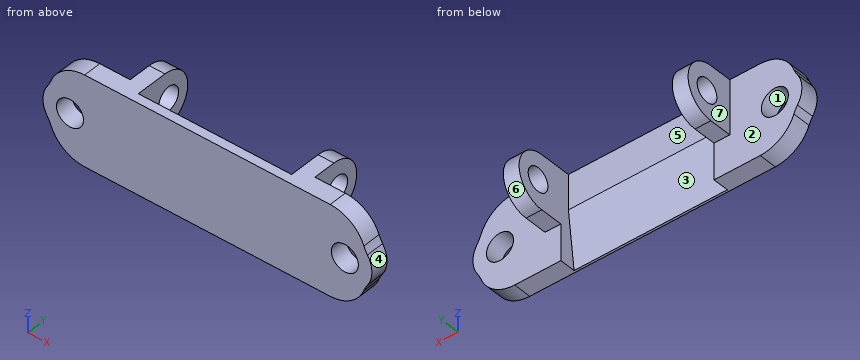
from build123d import *

# Parameters (mm, degrees)
BOSS_EXTRUDE1_DEPTH             = 4
CUT_EXTRUDE1_DEPTH              = 34
BOSS_EXTRUDE2_DEPTH             = 3.5
F_5_2_5_2_DIAMETER_HOLE1_REACH  = 64.241
F_5_2_5_2_DIAMETER_HOLE1_BORE_R = 2.6
F_6_0_6_DIAMETER_HOLE1_D        = 6
F_6_0_6_DIAMETER_HOLE1_DEPTH    = 15


with BuildPart() as part:
    # Sketch1 → Boss-Extrude1 (new body)
    with BuildSketch(Plane(origin=(0, 4, 0), x_dir=(1, 0, 0), z_dir=(0, 1, 0))):
        with BuildLine():
            Line((7.753999476, 0), (62.246000524, 0))
            ThreePointArc((62.246000524, 0), (66.787860981, 1.414295513), (69.723838222, 5.157124101))
            ThreePointArc((69.723838222, 5.157124101), (70.077199101, 5.953180748), (70.515003965, 6.706106372))
            ThreePointArc((70.515003965, 6.706106372), (71.5, 10), (70.515003965, 13.293893628))
            ThreePointArc((70.515003965, 13.293893628), (70.077199101, 14.046819252), (69.723838222, 14.842875899))
            ThreePointArc((69.723838222, 14.842875899), (66.787860981, 18.585704487), (62.246000524, 20))
            Line((62.246000524, 20), (52, 20))
            add(Edge.make_bspline(
                [(18, 20), (29.333333333, 20), (40.666666667, 20), (52, 20)],
                knots=[0, 0, 0, 0, 1, 1, 1, 1], degree=3))
            Line((18, 20), (7.753999476, 20))
            ThreePointArc((7.753999476, 20), (3.212139019, 18.585704487), (0.276161778, 14.842875899))
            ThreePointArc((0.276161778, 14.842875899), (-0.077199101, 14.046819252), (-0.515003965, 13.293893628))
            ThreePointArc((-0.515003965, 13.293893628), (-1.5, 10), (-0.515003965, 6.706106372))
            ThreePointArc((-0.515003965, 6.706106372), (-0.077199101, 5.953180748), (0.276161778, 5.157124101))
            ThreePointArc((0.276161778, 5.157124101), (3.212139019, 1.414295513), (7.753999476, 0))
        make_face()
    extrude(amount=-BOSS_EXTRUDE1_DEPTH)

    # Sketch2 → Cut-Extrude1 (cut)
    with BuildSketch(Plane(origin=(18, 0, 0), x_dir=(0, -1, 0), z_dir=(-1, 0, 0))):
        Polygon((-2, 0), (-4, 0), (-4, -20), (-0.499398694, -20), (-2, -7.707188193), align=None)
    extrude(amount=-CUT_EXTRUDE1_DEPTH, mode=Mode.SUBTRACT)

    # Sketch3 → Boss-Extrude2 (add)
    with BuildSketch(Plane(origin=(18, 0, 0), x_dir=(0, 0, -1), z_dir=(1, 0, 0))):
        with BuildLine():
            Line((0, 4), (12, 4))
            Line((12, 4), (12, 9))
            ThreePointArc((12, 9), (6, 15), (0, 9))
            Line((0, 9), (0, 4))
        make_face()
    boss_extrude2 = extrude(amount=-BOSS_EXTRUDE2_DEPTH)

    # Mirror1: Boss-Extrude2 across plane
    add(boss_extrude2.mirror(Plane.ZY.offset(-35)))

    # Ø5.2 (5.2) Diameter Hole1 bore → Ø5.2 (5.2) Diameter Hole1 (cut, up to next)
    with BuildSketch(Plane.ZY.offset(-14.5), mode=Mode.PRIVATE) as f_5_2_5_2_diameter_hole1_sk1:
        with Locations((-6, 10)):
            Circle(F_5_2_5_2_DIAMETER_HOLE1_BORE_R)
    f_5_2_5_2_diameter_hole1_tool1 = extrude(f_5_2_5_2_diameter_hole1_sk1.sketch, amount=-F_5_2_5_2_DIAMETER_HOLE1_REACH, mode=Mode.PRIVATE) & part.part
    f_5_2_5_2_diameter_hole1 = f_5_2_5_2_diameter_hole1_tool1.solids().sort_by_distance((14.5, 10, -6))[0]
    add(f_5_2_5_2_diameter_hole1, mode=Mode.SUBTRACT)

    # Ø6.0 (6) Diameter Hole1
    with Locations(Plane(origin=(0, 0, 0), x_dir=(-1, 0, 0), z_dir=(0, -1, 0))):
        with Locations((-4.5, 10)):
            f_6_0_6_diameter_hole1 = Hole(F_6_0_6_DIAMETER_HOLE1_D / 2, depth=F_6_0_6_DIAMETER_HOLE1_DEPTH)

    # Mirror2: Ø5.2 (5.2) Diameter Hole1, Ø6.0 (6) Diameter Hole1 across plane
    add(f_5_2_5_2_diameter_hole1.mirror(Plane.ZY.offset(-35)), mode=Mode.SUBTRACT)
    add(f_6_0_6_diameter_hole1.mirror(Plane.ZY.offset(-35)), mode=Mode.SUBTRACT)


solid = part.part
Could you check a few things on this model? Use its own coordinates, in mm. Face numbers are marked on the shaded views. A direction names the side the tool comes from. Give positions to 0.01 mm unless a question says otherwise; leave off trailing zeros. Order: outer loops, then holes, each group sorted by start corner. A loop starts at its lowest first (then second) coordinate and runs counter-clockwise, first axis right, second up.
1. We'd pull the mould along Z, two halves only. Please class the marked faces 1, 2, 3 and 4: pulls with the +Z half, pulls with the -Z half, needs draft (parallel to the pull), parting line crosses it, or undercut.
2. Suppose I cut it at C-C (x = 15.5). List the corners of the cut face in (y, z) for me.
3. Suppose I cut it at A-A (y = 5). List the corners of the cut face in (x, z) for me, plus the area to 3 significant figures.
4. Suppose I cut it at D-D (y = 10). List the corners of the cut face in (x, z) for me, plus the area to 3 significant figures.
5. For the marked faces 5, 6 and 7, which set-ups out of +Z, -Z, +X, -X, +Y, -Y let a thin tool reach every point of the face, with its end or its side?
6. Suppose I cut it at B-B (z = -6). List the corners of the cut face in (x, y) for me, plus the area to 3 significant figures.
7. Will these pins go through, and if not, where does the flat tip stop? P1, Ø3.5, axis at y = 9, z = -6, coming from the -X side; P2, Ø1, axis at x = 16, y = 6.5, coming from the -Z side; P3, Ø3.5, axis at y = 7, z = -5.5, coming from the +X side.
8. I need wall thicknesses on L1, parallel to X at y = 12.5, z = -7; L2, parallel to X at y = 3.75, z = -12.5; L3, parallel to Y at x = 62.5, z = -1.25. Which ranges of each line are inside material? Lowest first, please.
Solved:
1. face 1: undercut
1. face 2: needs draft
1. face 3: pulls with the -Z half
1. face 4: parting line crosses it
2. outline: (0, -20) - (4, -20) - (4, -12) - (9, -12) arc R6 ccw to (9, 0) - (0, 0) - close; hole circle Ø5.2 at (10, -6)
3. outline: (14.5, -12) - (18, -12) - (18, 0) - (14.5, 0) - close; (52, -12) - (55.5, -12) - (55.5, 0) - (52, 0) - close
3. area: 84.0 mm2
4. outline: (14.5, -11.92) - (18, -11.92) - (18, -8.6) - (14.5, -8.6) - close; (14.5, -3.4) - (18, -3.4) - (18, -0.08) - (14.5, -0.08) - close; (52, -11.92) - (55.5, -11.92) - (55.5, -8.6) - (52, -8.6) - close; (52, -3.4) - (55.5, -3.4) - (55.5, -0.08) - (52, -0.08) - close
4. area: 46.4 mm2
5. face 5: +Z, -Z, +Y
5. face 6: +X, -X, +Y
5. face 7: +Z, -Z, -X, +Y
6. outline: (-0.1, 0) - (70.1, 0) - (70.1, 4) - (55.5, 4) - (55.5, 7.4) - (52, 7.4) - (52, 2) - (18, 2) - (18, 7.4) - (14.5, 7.4) - (14.5, 4) - (-0.1, 4) - close; (14.5, 12.6) - (18, 12.6) - (18, 15) - (14.5, 15) - close; (52, 12.6) - (55.5, 12.6) - (55.5, 15) - (52, 15) - close
6. area: 253 mm2
7. P1: stops at x = 14.5
7. P2: stops at z = -12
7. P3: stops at x = 55.5
8. L1: x = 14.5 to 18, 52 to 55.5
8. L2: x = -0.95 to 2.84, 6.16 to 18, 52 to 63.84, 67.16 to 70.95
8. L3: y = 0 to 4
